Geometry check sheet. Reference: the model listing, model coordinates, mm. A direction names the side the tool comes from. Give positions to 0.01 mm unless a question says otherwise; leave off trailing zeros. Order: outer loops, then holes, each group sorted by start corner. A loop starts at its lowest first (then second) coordinate and runs counter-clockwise, first axis right, second up.
```python
from build123d import *

# Parameters (mm, degrees)
BOSS_EXTRUDE1_DEPTH = 30
SKETCH4_W           = 24
SKETCH4_H           = 14
CUT_EXTRUDE2_DEPTH  = 25
SKETCH5_W           = 1.7
SKETCH5_H           = 1.8
CUT_EXTRUDE3_DEPTH  = 15
CUT_EXTRUDE4_DEPTH  = 11
BOSS_EXTRUDE2_DEPTH = 3
SKETCH8_R           = 1.25
BOSS_EXTRUDE3_DEPTH = 4
FILLET3_R           = 1


with BuildPart() as part:
    # Sketch1 → Boss-Extrude1 (new body)
    with BuildSketch(Plane.XY):
        Polygon((0, 0), (0, -28), (12, -28), (12, -18), (5, 0), align=None)
    extrude(amount=-BOSS_EXTRUDE1_DEPTH)

    # Sketch4 → Cut-Extrude2 (cut)
    with BuildSketch(Plane.ZY):
        with Locations((-15, -22.638599401)):
            Rectangle(SKETCH4_W, SKETCH4_H)
    extrude(amount=-CUT_EXTRUDE2_DEPTH, mode=Mode.SUBTRACT)

    # Sketch5 → Cut-Extrude3 (cut)
    with BuildSketch(Plane.ZY):
        with Locations((-2.15, -25.7)):
            Rectangle(SKETCH5_W, SKETCH5_H)
    cut_extrude3 = extrude(amount=-CUT_EXTRUDE3_DEPTH, mode=Mode.SUBTRACT)

    # Mirror1: Cut-Extrude3 across plane
    add(cut_extrude3.mirror(Plane.XY.offset(-15)), mode=Mode.SUBTRACT)

    # Sketch6 → Cut-Extrude4 (cut, symmetric)
    with BuildSketch(Plane.XY.offset(-15)):
        Polygon((5, 0), (5, -13), (10.055555556, -13), align=None)
    extrude(amount=CUT_EXTRUDE4_DEPTH, both=True, mode=Mode.SUBTRACT)

    # Sketch7 → Boss-Extrude2 (add)
    with BuildSketch(Plane(origin=(0, -15, 0), x_dir=(1, 0, 0), z_dir=(0, 1, 0))):
        Polygon((0, 15), (-3, 15), (-5.356060357, 18.232488143), (-8.356060357, 18.232488143), (-8.356060357, 15.232488143), (-6.881763998, 15.232488143), (-4.525703641, 12), (0, 12), align=None)
    extrude(amount=BOSS_EXTRUDE2_DEPTH)

    # Sketch8 → Boss-Extrude3 (add)
    with BuildSketch(Plane(origin=(0, -15, 0), x_dir=(-1, 0, 0), z_dir=(0, -1, 0))):
        with Locations(Location((6.856060357, 16.632488143, 0), (0, 0, 270))):
            Circle(SKETCH8_R)
    extrude(amount=BOSS_EXTRUDE3_DEPTH)

    # Fillet3
    fillet3_edges = [part.edges().sort_by_distance(p)[0] for p in [
        (-6.856060357, -19, -17.882488143),
    ]]
    fillet(fillet3_edges, radius=FILLET3_R)


solid = part.part
```
Q1. Cross-section at D-D, the plane x = 2.5. Record the boundary of the cut face in (y, z).
Q2. Release check for a two-part mould opening along X. For faces 6 (the face through (-8.356, -14, -17)), 7 (the face through (-1, -14, -15)), 8 (the face through (-4, -15, -14)), 9 (the face through (6, -28, -28)) record: pulls with the +X half, pulls with the -X half, needs draft (parallel to the pull), parting line crosses it, or undercut.
Q3. Cross-section at C-C, the plane y = -9. Record the boundary of the cut face in (x, z).
Q4. Cross-section at B-B, the plane y = -21.75. Record the boundary of the cut face in (x, z), and give its area (3 significant figures).
Q5. Gauge pin test, flat ends, axial feed: P1, Ø1.5, axis at x = 8, z = -16, coming from the -Y side; P2, Ø1.9, axis at x = -4, z = -13.5, coming from the +Y side; P3, Ø0.9, axis at x = -2.5, y = -14, coming from the +Z side; P4, Ø12, axis at x = 0.5, z = -4.5, coming from the -Y side. Record the tip position at first contact, or that the pin passes through.
Q6. Thickness scan on L1, parallel to Z at x = 5.25, y = -21; L2, parallel to X at y = -6.75, z = -12.25; L3, parallel to Y at x = 9.5, z = -9.25. Record the ranges inside material, lowest first.
Q7. Cross-section at A-A, the plane z = -1.75. Record the boundary of the cut face in (x, y), and give its area (3 significant figures).
Q8. Access from +Z, -Z, +X, -X, +Y, -Y to the whole of each face (thin tool, end or side, straight path). Record for faces 1 (the face through (5, -17, -30)), 2 (the face through (6, -26.6, -28)), 3 (the face through (7, -13, -15)), 4 (the face through (6, -20, -3)), 5 (the face through (-6.91, -16.48, -17.88)).
Answers follow:
1. outline: (-28, -30) - (0, -30) - (0, 0) - (-28, 0) - (-28, -3) - (-26.6, -3) - (-26.6, -1.3) - (-24.8, -1.3) - (-24.8, -3) - (-15.64, -3) - (-15.64, -27) - (-24.8, -27) - (-24.8, -28.7) - (-26.6, -28.7) - (-26.6, -27) - (-28, -27) - close
2. face 6: pulls with the -X half
2. face 7: undercut
2. face 8: undercut
2. face 9: needs draft
3. outline: (0, -30) - (8.5, -30) - (8.5, -26) - (5, -26) - (5, -4) - (8.5, -4) - (8.5, 0) - (0, 0) - close
4. outline: (0, -30) - (12, -30) - (12, -27) - (0, -27) - close; (0, -3) - (12, -3) - (12, 0) - (0, 0) - close
4. area: 72.0 mm2
5. P1: stops at y = -15.64
5. P2: stops at y = -12
5. P3: stops at z = -12
5. P4: stops at y = -28
6. L1: z = -30 to -27, -3 to 0
6. L2: x = 0 to 5
6. L3: y = -15.64 to -13
7. outline: (0, -28) - (12, -28) - (12, -26.6) - (0, -26.6) - close; (0, -24.8) - (12, -24.8) - (12, -18) - (5, 0) - (0, 0) - close
7. area: 251 mm2
8. face 1: -Z, +X, -X, +Y, -Y
8. face 2: +X, -X
8. face 3: +X, +Y
8. face 4: +X, -X, -Y
8. face 5: -Y
